from build123d import *

# Parameters (mm, degrees)
PAD_DEPTH       = 5
SKETCH001_R     = 1.5
POCKET_DEPTH    = 5.001
SKETCH002_R     = 3
POCKET001_DEPTH = 3


with BuildPart() as part:
    # Sketch → Pad (new body)
    with BuildSketch(Plane.XZ):
        Polygon((0, 0), (0, 54.75), (10, 54.75), (76, 10), (76, 0), align=None)
    extrude(amount=PAD_DEPTH)

    # Sketch001 (on Face7 of Pad) → Pocket (cut, through all)
    with BuildSketch(Plane.XZ.offset(5)):
        with Locations((5, 51)):
            Circle(SKETCH001_R)
        with Locations((5, 43.5)):
            Circle(SKETCH001_R)
        with Locations((5, 28.5)):
            Circle(SKETCH001_R)
        with Locations((71, 5)):
            Circle(SKETCH001_R)
    extrude(amount=-POCKET_DEPTH, mode=Mode.SUBTRACT)

    # Sketch002 (on Face5 of Pocket) → Pocket001 (cut)
    with BuildSketch(Plane.XZ.offset(5)):
        with Locations((5, 51)):
            Circle(SKETCH002_R)
        with Locations((5, 43.5)):
            Circle(SKETCH002_R)
        with Locations((5, 28.5)):
            Circle(SKETCH002_R)
        with Locations((71, 5)):
            Circle(SKETCH002_R)
    extrude(amount=-POCKET001_DEPTH, mode=Mode.SUBTRACT)


solid = part.part
Model file for the job. Use its own axes, mm. A direction names the side the tool comes from. Give positions to 0.01 mm unless a question says otherwise; leave off trailing zeros. Order: outer loops, then holes, each group sorted by start corner. A loop starts at its lowest first (then second) coordinate and runs counter-clockwise, first axis right, second up. Notation, with made-up numbers: M 44,51.25 L 80,51.25 A14 cw 80,68.25 Z; hole C -23.5,35 d2. An arc over 180 degrees is marked long. Write item = value, one per line.
Q1. Drill centre lines: line 1 (Z direction, x = 5, y = -3.9); line 2 (Z direction, x = 5, y = -0.9); line 3 (Z direction, x = 31, y = -1.6). Where is each one in solid material? Low to high. Write a range as [from, to].
Derived:
line_1 = [0, 25.5], [31.5, 40.5], [46.5, 48], [54, 54.75]
line_2 = [0, 27], [30, 42], [45, 49.5], [52.5, 54.75]
line_3 = [0, 40.51]
Q2. Cut at B-B, the plane y = -1.2. List the corners of the cut face in (x, z), then the cut area to 3 significant figures.
Derived:
outline = M 0,0 L 76,0 L 76,10 L 10,54.75 L 0,54.75 Z; hole C 5,28.5 d3; hole C 5,43.5 d3; hole C 5,51 d3; hole C 71,5 d3
area = 2,660 mm2
Q3. Cut at C-C, the plane z = 28.5. List the corners of the cut face in (x, y).
Derived:
outline = M 0,-5 L 2,-5 L 2,-2 L 3.5,-2 L 3.5,0 L 0,0 Z; M 6.5,-2 L 8,-2 L 8,-5 L 48.72,-5 L 48.72,0 L 6.5,0 Z
Q4. Two-plate mould, pull along Z, no slides. Class faces 3 (the cylindrical face through (5, -1, 42)), 4 (the cylindrical face through (4.675, -1.014, 49.536)), 5 (the flat face through (30, 0, 22)), 6 (the flat face through (5, -2, 54.75)): pulls with the +Z half, pulls with the -Z half, needs draft (parallel to the pull), parting line crosses it, or undercut.
Derived:
face_3 = undercut
face_4 = undercut
face_5 = needs draft
face_6 = pulls with the +Z half
Q5. Cut at A-A, the plane z = 5. List the corners of the cut face in (x, y).
Derived:
outline = M 0,-5 L 68,-5 L 68,-2 L 69.5,-2 L 69.5,0 L 0,0 Z; M 72.5,-2 L 74,-2 L 74,-5 L 76,-5 L 76,0 L 72.5,0 Z
Q6. Flat gauge pins, fed straight in: pin 1 (3.5 mm diameter, centred on x = 5, z = 43.5, fed in from -Y); pin 2 (2.5 mm diameter, centred on x = 5, z = 51, fed in from -Y); pin 3 (1 mm diameter, centred on x = 20.5, y = -3.5, fed in from +Z). Where does each tip first touch, or does it go through?
Derived:
pin_1 = -2
pin_2 = through
pin_3 = 47.97
Q7. Cut at D-D, the plane x = 46. List the corners of the cut face in (y, z), then the cut area to 3 significant figures.
Derived:
outline = M -5,0 L 0,0 L 0,30.34 L -5,30.34 Z
area = 152 mm2
Q8. Tool access for faces 1 (the flat face through (6, -2, 45)), 2 (the cylindrical face through (72.43, -1.01, 5.45)): list every direction of +Z, -Z, +X, -X, +Y, -Y with a clear straight run to the whole face (end or side of a thin tool).
Derived:
face_1 = -Y
face_2 = +Y, -Y
